Answer from the drawing. Dimensions are ordinates in mm from the lowest x, y and z of the part. Give positions to 0.01 mm unless a question says otherwise; leave off trailing zeros. Write each loop counter-clockwise with the first axis right and the second up, starting at its lowest first coordinate (ties: lowest second). Pieces come first, ordered by that corner, then holes.
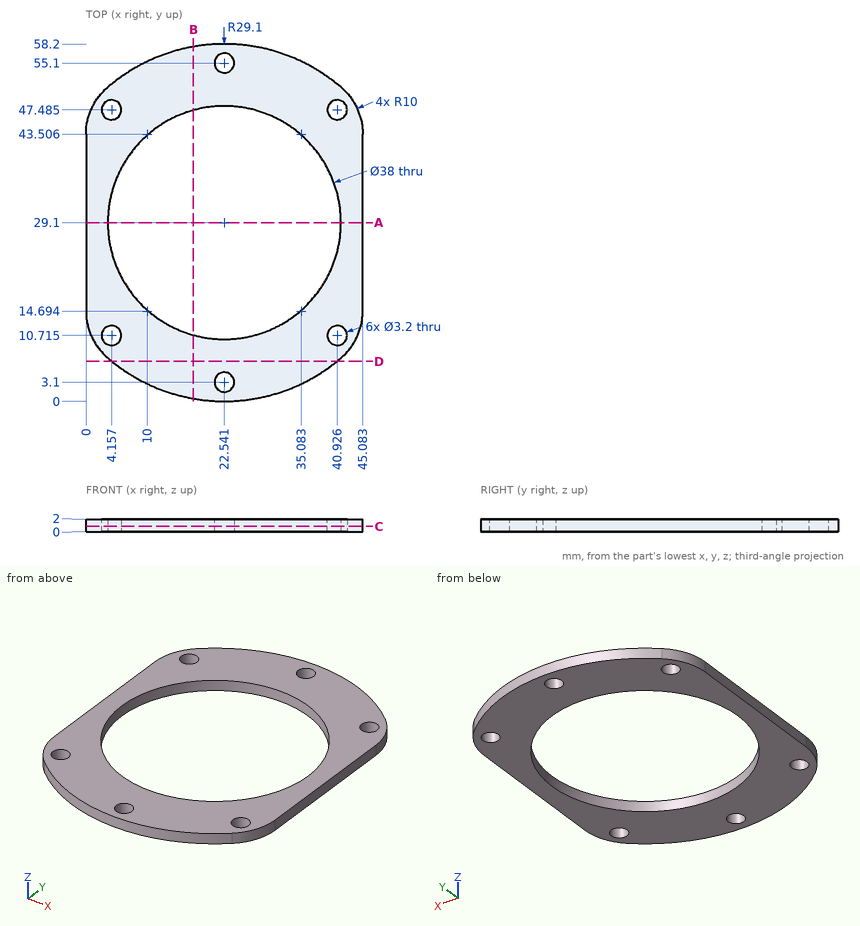
Item 1: A cutting plane is placed at B-B, the plane x = 17.5. Give the vertices of the cut face in (y, z).
Conclusion:
outline: (0.44, 0) - (10.78, 0) - (10.78, 2) - (0.44, 2) - close; (47.42, 0) - (57.76, 0) - (57.76, 2) - (47.42, 2) - close
Item 2: A cutting plane is placed at A-A, the plane y = 29.1. Give the vertices of the cut face in (x, z).
Conclusion:
outline: (0, 0) - (3.54, 0) - (3.54, 2) - (0, 2) - close; (41.54, 0) - (45.08, 0) - (45.08, 2) - (41.54, 2) - close
Item 3: A cutting plane is placed at D-D, the plane y = 6.5. Give the vertices of the cut face in (x, z).
Conclusion:
outline: (4.21, 0) - (40.87, 0) - (40.87, 2) - (4.21, 2) - close
Item 4: Consider probe 1 along X at (y, z) = (48.5, 1.4) (1 decimal); probe 2 along X at (y, z) = (27, 1.25) (1 decimal); probe 3 along Y at (x, z) = (9, 0.8) (1 decimal). Determine where each line is inside the solid, lowest interval first.
Conclusion:
probe 1: x = 1.3 to 2.9, 5.4 to 39.7, 42.2 to 43.7
probe 2: x = 0 to 3.7, 41.4 to 45.1
probe 3: y = 3.3 to 15.8, 42.4 to 54.9
Item 5: A cutting plane is placed at C-C, the plane z = 0.85. Give the vertices of the cut face in (x, y) (1 decimal), plus the area to 3 significant figures.
Conclusion:
outline: (0, 14.7) arc R10 ccw to (3.4, 7.2) arc R29.1 ccw to (41.6, 7.2) arc R10 ccw to (45.1, 14.7) - (45.1, 43.5) arc R10 ccw to (41.6, 51) arc R29.1 ccw to (3.4, 51) arc R10 ccw to (0, 43.5) - close; hole circle Ø3.2 at (4.2, 10.7); hole circle Ø3.2 at (4.2, 47.5); hole circle Ø38 at (22.5, 29.1); hole circle Ø3.2 at (22.5, 3.1); hole circle Ø3.2 at (22.5, 55.1); hole circle Ø3.2 at (40.9, 10.7); hole circle Ø3.2 at (40.9, 47.5)
area: 1,140 mm2
Item 6: Each of these flat-tipped pins is pushed along its axis until it touches: P1, Ø5, axis at x = 40.93, y = 10.72, coming from the +Z side; P2, Ø23, axis at x = 22.54, y = 29.1, coming from the +Z side. Where does it stop, or does it pass through?
Conclusion:
P1: stops at z = 2
P2: passes through
